from build123d import *

# Parameters (mm, degrees)
F0_W     = 20.82
F0_H     = 5
F1_DEPTH = 8.5
F2_W     = 1.5
F2_H     = 1.5
F3_DEPTH = 7
F4_W     = 0.6
F4_H     = 0.4
F5_DEPTH = 3


with BuildPart() as f1:
    # F0 (on Top) → F1 (new body)
    with BuildSketch(Plane.XY):
        Rectangle(F0_W, F0_H)
    extrude(amount=F1_DEPTH)

    # F2 (on face) → F3 (cut)
    with BuildSketch(Plane.XY.offset(8.5)):
        with Locations((-8.89, 1.27)):
            Rectangle(F2_W, F2_H)
        with Locations((-8.89, -1.27)):
            Rectangle(F2_W, F2_H)
        with Locations((-6.35, 1.27)):
            Rectangle(F2_W, F2_H)
        with Locations((-6.35, -1.27)):
            Rectangle(F2_W, F2_H)
        with Locations((-3.81, 1.27)):
            Rectangle(F2_W, F2_H)
        with Locations((-3.81, -1.27)):
            Rectangle(F2_W, F2_H)
        with Locations((-1.27, 1.27)):
            Rectangle(F2_W, F2_H)
        with Locations((-1.27, -1.27)):
            Rectangle(F2_W, F2_H)
        with Locations((1.27, 1.27)):
            Rectangle(F2_W, F2_H)
        with Locations((1.27, -1.27)):
            Rectangle(F2_W, F2_H)
        with Locations((3.81, 1.27)):
            Rectangle(F2_W, F2_H)
        with Locations((3.81, -1.27)):
            Rectangle(F2_W, F2_H)
        with Locations((6.35, 1.27)):
            Rectangle(F2_W, F2_H)
        with Locations((6.35, -1.27)):
            Rectangle(F2_W, F2_H)
        with Locations((8.89, 1.27)):
            Rectangle(F2_W, F2_H)
        with Locations((8.89, -1.27)):
            Rectangle(F2_W, F2_H)
    extrude(amount=-F3_DEPTH, mode=Mode.SUBTRACT)

    # F4 (on face) → F5 (join)
    with BuildSketch(Plane(origin=(0, 0, 0), x_dir=(1, 0, 0), z_dir=(0, 0, -1))):
        with Locations((-8.89, 1.27)):
            Rectangle(F4_W, F4_H)
        with Locations((-8.89, -1.27)):
            Rectangle(F4_W, F4_H)
        with Locations((-6.35, 1.27)):
            Rectangle(F4_W, F4_H)
        with Locations((-6.35, -1.27)):
            Rectangle(F4_W, F4_H)
        with Locations((-3.81, 1.27)):
            Rectangle(F4_W, F4_H)
        with Locations((-3.81, -1.27)):
            Rectangle(F4_W, F4_H)
        with Locations((-1.27, 1.27)):
            Rectangle(F4_W, F4_H)
        with Locations((-1.27, -1.27)):
            Rectangle(F4_W, F4_H)
        with Locations((1.27, 1.27)):
            Rectangle(F4_W, F4_H)
        with Locations((1.27, -1.27)):
            Rectangle(F4_W, F4_H)
        with Locations((3.81, 1.27)):
            Rectangle(F4_W, F4_H)
        with Locations((3.81, -1.27)):
            Rectangle(F4_W, F4_H)
        with Locations((6.35, 1.27)):
            Rectangle(F4_W, F4_H)
        with Locations((6.35, -1.27)):
            Rectangle(F4_W, F4_H)
        with Locations((8.89, 1.27)):
            Rectangle(F4_W, F4_H)
        with Locations((8.89, -1.27)):
            Rectangle(F4_W, F4_H)
    extrude(amount=F5_DEPTH)


solid = f1.part
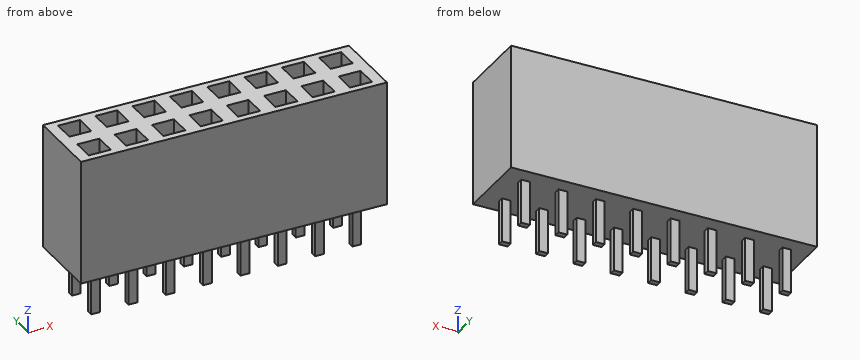
Here's how the part is built. I have some questions about the finished solid (model axes, mm). Give positions to 0.01 mm unless a question says otherwise; leave off trailing zeros. Order: outer loops, then holes, each group sorted by start corner. A loop starts at its lowest first (then second) coordinate and runs counter-clockwise, first axis right, second up. Notation, with made-up numbers: (25.5, -10.75) -> (52.5, -10.75) arc R24 ccw to (52.5, 25.25) -> close; hole circle Ø8 at (69, -2.75). An arc over 180 degrees is marked (long way). One line per item, written item: value. Start each with the question number.
1. Imagine slicing it at A-A, the plane x = 1.25. List the corners of the cut face in (y, z) for me, plus the area to 3 significant figures.
2. Imagine slicing it at D-D, the plane x = -5.25. List the corners of the cut face in (y, z) for me, plus the area to 3 significant figures.
3. Imagine slicing it at C-C, the plane z = 3.5. Count the separate pieces of the cut face and the enclosed holes in it, plus the area to 3 significant figures.
4. Will this pin go through, and if not, where does the flat tip stop? pin 1 Ø0.5 at (x, z) = (-1.5, -2) entering from -Y.
5. I need wall thicknesses on probe 1 along Y at (x, z) = (-4.25, 2.75); probe 2 along Y at (x, z) = (-1.5, -1.75); probe 3 along Z at (x, y) = (-9, 0.1). Which ranges of each line are inside material? Lowest first, please. Write a range as from..to.
6. Imagine slicing it at B-B, the plane y = 0.2. List the corners of the cut face in (x, z) for me, plus the area to 3 significant figures.
Values follow:
1. outline: (-2.5, 0) -> (-1.47, 0) -> (-1.47, -3) -> (-1.07, -3) -> (-1.07, 0) -> (1.07, 0) -> (1.07, -3) -> (1.47, -3) -> (1.47, 0) -> (2.5, 0) -> (2.5, 8.5) -> (2.02, 8.5) -> (2.02, 1.5) -> (0.52, 1.5) -> (0.52, 8.5) -> (-0.52, 8.5) -> (-0.52, 1.5) -> (-2.02, 1.5) -> (-2.02, 8.5) -> (-2.5, 8.5) -> close
1. area: 23.9 mm2
2. outline: (-2.5, 0) -> (2.5, 0) -> (2.5, 8.5) -> (-2.5, 8.5) -> close
2. area: 42.5 mm2
3. separate pieces: 1
3. enclosed holes: 16
3. area: 68.1 mm2
4. pin 1: stops at y = -1.47
5. probe 1: y = -2.5..-2.02, -0.52..0.52, 2.02..2.5
5. probe 2: y = -1.47..-1.07, 1.07..1.47
5. probe 3: z = 0..8.5
6. outline: (-10.41, 0) -> (10.41, 0) -> (10.41, 8.5) -> (-10.41, 8.5) -> close
6. area: 177 mm2
